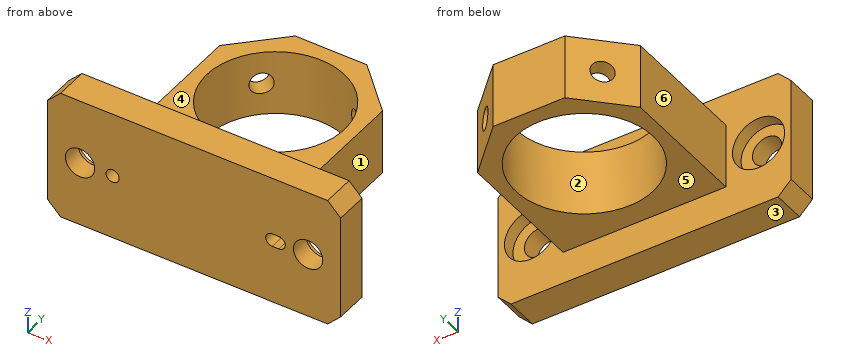
Autodesk Inventor part; units mm, degrees
ref_plane "YZ Plane" through (0, 0, 0) normal (1, 0, 0) x (0, 1, 0)
ref_plane "XZ Plane" through (0, 0, 0) normal (0, 1, 0) x (-1, 0, 0)
ref_plane "XY Plane" through (0, 0, 0) normal (0, 0, 1) x (1, 0, 0)
sketch "Sketch2" plane through (0, 0, 0) normal (0, 1, 0) x (-1, 0, 0)
  line L0 (-22.5, 10) -> (22.5, 10)
  line L1 (22.5, 10) -> (22.5, -10)
  line L2 (22.5, -10) -> (-22.5, -10)
  line L3 (-22.5, -10) -> (-22.5, 10)
  line L4 (-22.5, 10) -> (22.5, -10) construction
  line L5 (22.5, 10) -> (-22.5, -10) construction
  point P0 (0, 0)
  dimension "d0" = 45
  dimension "d1" = 20
extrude "Extrusion1" add sketch "Sketch2" along normal blind 5
sketch "Sketch3" plane through (0, 5, 0) normal (0, 1, 0) x (1, 0, 0)
  line L0 (12.5, -5) -> (-12.5, -5)
  line L1 (-12.5, -5) -> (-12.5, 5)
  line L2 (-12.5, 5) -> (12.5, 5)
  line L3 (12.5, 5) -> (12.5, -5)
  line L4 (12.5, -5) -> (-12.5, 5) construction
  line L5 (-12.5, -5) -> (12.5, 5) construction
  point P0 (0, 0)
  dimension "d4" = 25
  dimension "d5" = 10
extrude "Extrusion2" add sketch "Sketch3" along normal blind 27
sketch "Sketch4" plane through (12.5, 5, -5) normal (0, 0, -1) x (-1, 0, 0)
  line L0 (35, 0) -> (-10, 0) construction
  line L1 (12.5, 0) -> (12.5, 14.05) construction
  circle A0 centre (12.5, 14.05) radius 10.55
  point P0 (12.5, -5)
  dimension "d8" = 14.05
  dimension "d9" = 21.1
extrude "Extrusion3" cut sketch "Sketch4" against normal up to surface (10 mm away)
chamfer "Chamfer1" distance 7 angle 45 2 edges at (12.5, 32, 0) (-12.5, 32, 0)
sketch "Sketch6" plane through (5.5, 32, -5) normal (0.7071, 0.7071, 0) x (-0.7071, 0.7071, 0)
  line L0 (0, 0) -> (0, 10) construction
  line L1 (-9.8995, 10) -> (-9.8995, 0) construction
  line L2 (0, 10) -> (-9.8995, 0) construction
  line L3 (-9.8995, 0) -> (-9.8995, 10) construction
  line L4 (-9.8995, 10) -> (0, 0) construction
  line L5 (0, 0) -> (-4.9497, 5) construction
  point P0 (-18.7383, 5)
hole "Hole1" at (9, 28.5, 0) direction (-0.7071, -0.7071, 0) diameter 3.302 depth 12.3
sketch "Sketch7" plane through (-5.5, 32, -5) normal (-0.7071, 0.7071, 0) x (-0.7071, -0.7071, 0)
  line L0 (0, 10) -> (0, 0) construction
  line L1 (24.0416, 0) -> (9.8995, 0) construction
  line L2 (0, 10) -> (9.8995, 0) construction
  line L3 (9.8995, 0) -> (4.9497, 5) construction
  point P0 (18.7383, 5)
hole "Hole2" at (-9, 28.5, 0) direction (0.7071, -0.7071, 0) diameter 3.302 depth 12.3
sketch "Sketch13" plane through (0, 5, 0) normal (0, 1, 0) x (1, 0, 0)
  line L0 (-22.5, 10) -> (-22.5, -10) construction
  line L1 (-22.5, 0) -> (-17.5, 0) construction
  line L2 (22.5, -10) -> (22.5, 10) construction
  line L3 (22.5, 0) -> (17.5, 0) construction
  circle A0 centre (17.5, 0) radius 4
  circle A1 centre (-17.5, 0) radius 4
  point P0 (0, 0)
  dimension "d69" = 5
  dimension "d70" = 5
  dimension "d71" = 8
  dimension "d72" = 8
extrude "Extrusion8" cut sketch "Sketch13" against normal blind 2
sketch "Sketch14" plane through (0, 5, 0) normal (0, 1, 0) x (1, 0, 0)
  circle A0 centre (17.5, 0) radius 4
  circle A1 centre (17.5, 0) radius 2.25
  circle A2 centre (-17.5, 0) radius 4
  circle A3 centre (-17.5, 0) radius 2.25
  point P0 (0, 0)
  dimension "d75" = 4.5
extrude "Extrusion9" cut sketch "Sketch14" against normal through all contours A1 | A3
sketch "Sketch15" plane through (0, 0, 0) normal (0, -1, 0) x (1, 0, 0)
  circle A0 centre (-17.5, 0) radius 2.25 construction
  line L0 (-17.5, 0) -> (-12.5, 0) construction
  circle A1 centre (17.5, 0) radius 2.25 construction
  line L1 (17.5, 0) -> (13, 0) construction
  circle A2 centre (-12.5, 0) radius 1.005
  circle A3 centre (13, 0) radius 1.005
  line L2 (13, 0) -> (12, 0) construction
  circle A4 centre (12, 0) radius 1.005
  line L3 (12, 1.005) -> (13, 1.005)
  line L4 (13, -1.005) -> (12, -1.005)
  point P0 (0, 0)
  dimension "d78" = 5
  dimension "d79" = 4.5
  dimension "d80" = 2.01
  dimension "d81" = 2.01
  dimension "d82" = 1
  dimension "d83" = 2.01
extrude "Extrusion10" cut sketch "Sketch15" against normal blind 2.1
chamfer "Chamfer3" distance 2 angle 45 4 edges at (-22.5, 2.5, 10) (22.5, 2.5, 10) (-22.5, 2.5, -10) (22.5, 2.5, -10)
properties part number "ADAPTER_I-355-03"
Model file for the job. Use its own axes, mm. Face numbers are marked on the shaded views. A direction names the side the tool comes from. Coordinates: 2 decimals unless noted, no trailing zeros. Order: outer loops, then holes, each group sorted by start corner. A loop starts at its lowest first (then second) coordinate and runs counter-clockwise, first axis right, second up. Notation, with made-up numbers: (68, -17) -> (94, -17) arc R5 ccw to (94, -13) -> close; hole circle Ø3 at (-10.75, -19). An arc over 180 degrees is marked (long way). Return JSON: item names as keys, results as strings. Group by question number.
Item 1: Saw through at B-B on x = -17.5. Write the cut outline in (y, z).
Item 2: Saw through at C-C on y = 4. Write the cut outline in (x, z), then the cut area to 3 significant figures.
Item 3: Wall check: line 1 along X through (y, z) = (4.4, 0); line 2 along Z through (x, y) = (17.5, 4.55); line 3 along X through (y, z) = (2.15, 0). Give the ranges that are in metal, low to high. Write a range as [from, to].
Item 4: Pull direction X, two halves, no side cores. Call the marked faces 1, 2 and 3: pulls with the +X half, pulls with the -X half, needs draft (parallel to the pull), parting line crosses it, or undercut.
Item 5: Tool access for the marked faces 4, 5 and 6: list every direction of +Z, -Z, +X, -X, +Y, -Y with a clear straight run to the whole face (end or side of a thin tool).
Item 6: Saw through at D-D on z = 3. Write the cut outline in (x, y).
Item 7: Saw through at A-A on y = 19.05. Write the cut outline in (x, z).
Item 8: Flat gauge pins, fed straight in: P1, Ø1.6, axis at x = -12.5, z = 0, coming from the +Y side; P2, Ø1.5, axis at x = -0.5, z = 6.5, coming from the +Y side; P3, Ø5, axis at y = 13, z = 0, coming from the +X side. Where does each tip first touch, or does it go through?
Values found:
{
 "1": {"outline": "(0, -10) -> (5, -10) -> (5, -4) -> (3, -4) -> (3, -2.25) -> (0, -2.25) -> close; (0, 2.25) -> (3, 2.25) -> (3, 4) -> (5, 4) -> (5, 10) -> (0, 10) -> close"},
 "2": {"outline": "(-22.5, -8) -> (-20.5, -10) -> (20.5, -10) -> (22.5, -8) -> (22.5, 8) -> (20.5, 10) -> (-20.5, 10) -> (-22.5, 8) -> close; hole circle Ø8 at (-17.5, 0); hole circle Ø8 at (17.5, 0)", "area": "791 mm2"},
 "3": {"line 1": "x = [-22.5, -21.5], [-13.5, 13.5], [21.5, 22.5]", "line 2": "z = [-10, -4], [4, 10]", "line 3": "x = [-22.5, -19.75], [-15.25, 15.25], [19.75, 22.5]"},
 "4": {"face 1": "pulls with the +X half", "face 2": "undercut", "face 3": "needs draft"},
 "5": {"face 4": "+Z, +X, -X, +Y", "face 5": "-Z, +X, -X, +Y", "face 6": "+Z, -Z, -X, +Y"},
 "6": {"outline": "(-22.5, 0) -> (22.5, 0) -> (22.5, 5) -> (20.15, 5) -> (20.15, 3) -> (14.85, 3) -> (14.85, 5) -> (12.5, 5) -> (12.5, 25) -> (5.5, 32) -> (-5.5, 32) -> (-12.5, 25) -> (-12.5, 5) -> (-14.85, 5) -> (-14.85, 3) -> (-20.15, 3) -> (-20.15, 5) -> (-22.5, 5) -> close; hole circle Ø21.1 at (0, 19.05)"},
 "7": {"outline": "(-12.5, -5) -> (-10.55, -5) -> (-10.55, 5) -> (-12.5, 5) -> close; (10.55, -5) -> (12.5, -5) -> (12.5, 5) -> (10.55, 5) -> close"},
 "8": {"P1": "stops at y = 25.8", "P2": "stops at y = 5", "P3": "stops at x = 12.5"}
}
